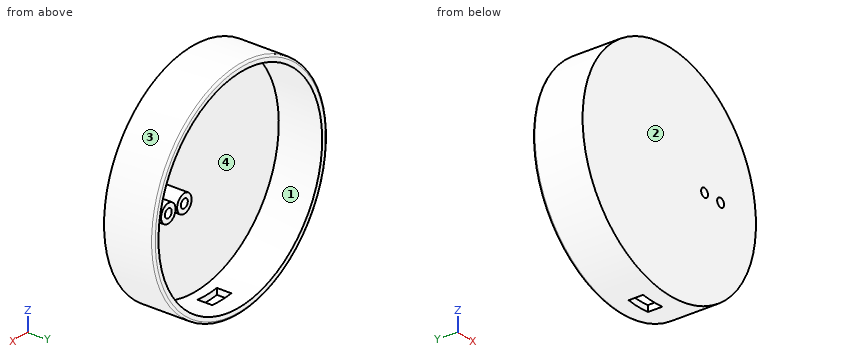
from build123d import *

# Parameters (mm, degrees)
SKETCH_1_R                     = 54
FLOOR_D108_T3_DEPTH            = 3
SKETCH_2_R                     = 54
SKETCH_2_R_2                   = 51
RIM_OD108_ID102_H24_DEPTH      = 24
SKETCH_3_R                     = 4.5
SENSOR_FIXED_POSTS_DEPTH       = 14
SKETCH_4_R                     = 2.15
M4_FIXED_MOUNT_CLEARANCE_DEPTH = 14
SKETCH_5_W                     = 12
SKETCH_5_H                     = 11
USB_C_SIDE_OPENING_12X7_DEPTH  = 7
BASE_OUTER_ROUND_R1_R          = 1


with BuildPart() as part:
    # 草图1 → Floor_D108_T3 (new body)
    with BuildSketch(Plane(origin=(0, 0, 0), x_dir=(1, 0, 0), z_dir=(0, 1, 0))):
        with Locations(Location((0, 0, 0), (0, 0, 270))):
            Circle(SKETCH_1_R)
    extrude(amount=FLOOR_D108_T3_DEPTH)

    # 草图2 → Rim_OD108_ID102_H24 (add)
    with BuildSketch(Plane(origin=(0, 0, 0), x_dir=(1, 0, 0), z_dir=(0, 1, 0))):
        with Locations(Location((0, 0, 0), (0, 0, 270))):
            Circle(SKETCH_2_R)
        with Locations(Location((0, 0, 0), (0, 0, 270))):
            Circle(SKETCH_2_R_2, mode=Mode.SUBTRACT)
    extrude(amount=RIM_OD108_ID102_H24_DEPTH)

    # 草图3 → Sensor_fixed_posts (add)
    with BuildSketch(Plane(origin=(0, 0, 0), x_dir=(1, 0, 0), z_dir=(0, 1, 0))):
        with Locations(Location((22, 0, 0), (0, 0, 270))):
            Circle(SKETCH_3_R)
        with Locations(Location((32, 0, 0), (0, 0, 270))):
            Circle(SKETCH_3_R)
    extrude(amount=SENSOR_FIXED_POSTS_DEPTH)

    # 草图4 → M4_fixed_mount_clearance (cut)
    with BuildSketch(Plane(origin=(0, 0, 0), x_dir=(1, 0, 0), z_dir=(0, 1, 0))):
        with Locations(Location((22, 0, 0), (0, 0, 270))):
            Circle(SKETCH_4_R)
        with Locations(Location((32, 0, 0), (0, 0, 270))):
            Circle(SKETCH_4_R)
    extrude(amount=M4_FIXED_MOUNT_CLEARANCE_DEPTH, mode=Mode.SUBTRACT)

    # 草图5 → USB_C_side_opening_12x7 (cut)
    with BuildSketch(Plane(origin=(0, 8, 0), x_dir=(1, 0, 0), z_dir=(0, 1, 0))):
        with Locations((0, 54.5)):
            Rectangle(SKETCH_5_W, SKETCH_5_H)
    extrude(amount=USB_C_SIDE_OPENING_12X7_DEPTH, mode=Mode.SUBTRACT)

    # Base_outer_round_R1
    base_outer_round_r1_edges = [part.edges().sort_by_distance(p)[0] for p in [
        (0, 24, -54),
    ]]
    fillet(base_outer_round_r1_edges, radius=BASE_OUTER_ROUND_R1_R)


solid = part.part
Could you check a few things on this model? Use its own coordinates, in mm. Face numbers are marked on the shaded views. Give positions to 0.01 mm unless a question says otherwise; leave off trailing zeros. Order: outer loops, then holes, each group sorted by start corner. A loop starts at its lowest first (then second) coordinate and runs counter-clockwise, first axis right, second up. Notation, with made-up numbers: (45.5, 12) - (103.5, 12) arc R22 cw to (103.5, 36) - close; hole circle Ø3 at (20.5, -10). An arc over 180 degrees is marked (long way). One line per question, with ' | ' between items. Start each with the question number.
Item 1: I want a section at B-B on z = 0. Write out the boundary of the cut face in (x, y).
Item 2: I'm going to push flat-ended pins straight in: pin 1 Ø4 at (x, z) = (29.5, -31.5) entering from +Y; pin 2 Ø10 at (x, z) = (21, 1.5) entering from +Y; pin 3 Ø8 at (x, y) = (-36.5, 20) entering from +Z. Where does each tip first touch, or does it pass through?
Item 3: Thinking about a two-plate mould opening in X: for the marked faces 1, 2, 3 and 4, which applies, pulls with the +X half, pulls with the -X half, needs draft (parallel to the pull), parting line crosses it, or undercut?
Item 4: I want a section at C-C on x = 0. Write out the boundary of the cut face in (y, z).
Item 5: I want a section at A-A on y = 12.5. Write out the boundary of the cut face in (x, z).
Item 6: I need wall thicknesses on probe 1 along X at (y, z) = (6.5, 0); probe 2 along Z at (x, y) = (0, 17.5); probe 3 along X at (y, z) = (13.75, -1.5). Which ranges of each line are inside material? Lowest first, please. Write a range as [from, to].
Verdict:
1) outline: (-54, 0) - (19.85, 0) - (19.85, 14) - (17.5, 14) - (17.5, 3) - (-51, 3) - (-51, 24) - (-53, 24) arc R1 ccw to (-54, 23) - close; (24.15, 0) - (29.85, 0) - (29.85, 14) - (27.5, 14) - (27.5, 3) - (26.5, 3) - (26.5, 14) - (24.15, 14) - close; (34.15, 0) - (54, 0) - (54, 23) arc R1 ccw to (53, 24) - (51, 24) - (51, 3) - (36.5, 3) - (36.5, 14) - (34.15, 14) - close
2) pin 1: y = 3 | pin 2: y = 14 | pin 3: z = 43.12
3) face 1: undercut | face 2: needs draft | face 3: parting line crosses it | face 4: undercut
4) outline: (0, -54) - (8, -54) - (8, -51) - (3, -51) - (3, 51) - (24, 51) - (24, 53) arc R1 ccw to (23, 54) - (0, 54) - close; (15, -54) - (23, -54) arc R1 ccw to (24, -53) - (24, -51) - (15, -51) - close
5) outline: (-6, -53.67) - (-6, -50.65) arc R51 cw (long way) to (6, -50.65) - (6, -53.67) arc R54 ccw (long way) to start; circle Ø9 at (22, 0); circle Ø9 at (32, 0); hole circle Ø4.3 at (22, 0); hole circle Ø4.3 at (32, 0)
6) probe 1: [-54, -51], [17.5, 19.85], [24.15, 26.5], [27.5, 29.85], [34.15, 36.5], [51, 54] | probe 2: [-54, -51], [51, 54] | probe 3: [-53.98, -50.98], [17.76, 20.46], [23.54, 26.24], [27.76, 30.46], [33.54, 36.24], [50.98, 53.98]
